from build123d import *

# Parameters (mm, degrees)
EXTRUDE_THIN1_DEPTH      = 10
EXTRUDE_THIN1_DEPTH_BACK = 25
SKETCH1_R                = 27.5
SKETCH1_R_2              = 22.5
CUT_EXTRUDE1_REACH       = 68.38
CUT_EXTRUDE1_END_RADIUS  = 22.5
SKETCH2_R                = 3.5
BOSS_EXTRUDE1_START      = -5
SKETCH3_R                = 22.5
BOSS_EXTRUDE1_DEPTH      = 5


with BuildPart() as part:
    # Sketch1 → Extrude-Thin1 (new, two sides: drawn at the far end of the back side and taken through both)
    with BuildSketch(Plane(origin=(0, 0, 0), x_dir=(1, 0, 0), z_dir=(0, 1, 0)).offset(-EXTRUDE_THIN1_DEPTH_BACK)):
        Circle(SKETCH1_R)
        Circle(SKETCH1_R_2, mode=Mode.SUBTRACT)
    extrude(amount=EXTRUDE_THIN1_DEPTH + EXTRUDE_THIN1_DEPTH_BACK)

    # Cut-Extrude1: up to this cylinder (the profile starts outside it)
    cut_extrude1_end = Plane(origin=(0, 0, 0), z_dir=(0, 1, 0)) * Cylinder(CUT_EXTRUDE1_END_RADIUS, 182.76, mode=Mode.PRIVATE)
    # Sketch2 → Cut-Extrude1 (cut, up to the surface)
    with BuildSketch(Plane.XY.offset(27.5), mode=Mode.PRIVATE) as cut_extrude1_sk1:
        with Locations(Location((0, 0, 0), (0, 0, 270))):
            Circle(SKETCH2_R)
    cut_extrude1_tool1 = extrude(cut_extrude1_sk1.sketch, amount=-CUT_EXTRUDE1_REACH, mode=Mode.PRIVATE) - cut_extrude1_end
    cut_extrude1 = cut_extrude1_tool1.solids().sort_by_distance((0, 0, 27.5))[0]
    add(cut_extrude1, mode=Mode.SUBTRACT)

    # Mirror1: Cut-Extrude1 across plane
    add(cut_extrude1.mirror(Plane.XY), mode=Mode.SUBTRACT)

    # Sketch3 → Boss-Extrude1 (add)
    with BuildSketch(Plane.XZ.offset(25).offset(BOSS_EXTRUDE1_START)):
        with Locations(Location((0, 0, 0), (0, 0, 90))):
            Circle(SKETCH3_R)
    extrude(amount=BOSS_EXTRUDE1_DEPTH)


solid = part.part
Can you work these out from the model? Positions are in its coordinate system, mm. A direction names the side the tool comes from. Round coordinates to 2 decimals unless told otherwise and drop trailing zeros. Order: outer loops, then holes, each group sorted by start corner. A loop starts at its lowest first (then second) coordinate and runs counter-clockwise, first axis right, second up. Notation, with made-up numbers: (-16, 23.25) - (26, 23.25) arc R25 cw to (26, 52.25) - close; hole circle Ø8 at (49, 82). An arc over 180 degrees is marked (long way). Answer in a Markdown table with one row per item.
(1) If we mould it in two halves opening along X, with no side actions, what happens to faces 3 (the face through (-5.961, -7.745, 26.846)), 4 (the face through (-3.417, 0.759, -24.9)), 5 (the face through (-23, 10, 0))? For each: released by +X, released by -X, zero draft, split by the parting line, or undercut.
From the geometry:
| item | result |
|---|---|
| face 3 | split by the parting line |
| face 4 | undercut |
| face 5 | zero draft |
(2) Suppose I cut it at B-B, the plane z = 0. Please give me the cut outline in (x, y), plus the area to 3 significant figures.
From the geometry:
| item | result |
|---|---|
| outline | (-27.5, -25) - (27.5, -25) - (27.5, 10) - (22.5, 10) - (22.5, -20) - (-22.5, -20) - (-22.5, 10) - (-27.5, 10) - close |
| area | 575 mm2 |
(3) Please list where these lines run through material, in increasing order: L1, parallel to Y at x = 0, z = -24; L2, parallel to Z at x = 0, y = -6; L3, parallel to X at y = -10, z = -14. Write a range as from..to.
From the geometry:
| item | result |
|---|---|
| L1 | y = -25..-3.5, 3.5..10 |
| L2 | z = -27.5..-22.5, 22.5..27.5 |
| L3 | x = -23.67..-17.61, 17.61..23.67 |
(4) Suppose I cut it at D-D, the plane y = -11. Please give me the cut outline in (x, z), plus the area to 3 significant figures.
From the geometry:
| item | result |
|---|---|
| outline | circle Ø55 at (0, 0); hole circle Ø45 at (0, 0) |
| area | 785 mm2 |
(5) For P1, Ø1, axis at y = -6.5, z = -13, coming from the +X side; P2, Ø2, axis at x = 10.5, z = 1.5, coming from the +Y side; P3, Ø8, axis at y = -15, z = 16.5, coming from the -X side; P4, Ø11, axis at x = 0, y = 0, coming from the -Z side, each with a flat end and sliding along its axis, tell me the tip position at first contact or that it passes through.
From the geometry:
| item | result |
|---|---|
| P1 | stops at x = 24.49 |
| P2 | stops at y = -20 |
| P3 | stops at x = -24.49 |
| P4 | stops at z = -27.5 |
(6) Which directions (+Z, -Z, +X, -X, +Y, -Y) give clear straight access to the entire face, cutting with the end or side of a thin tool? Please do faces 1 (the face through (-1.341, -3.233, 24.9)), 2 (the face through (-4.878, -5.21, 21.965)).
From the geometry:
| item | result |
|---|---|
| face 1 | +Z, -Z |
| face 2 | +Y |
(7) Suppose I cut it at A-A, the plane x = 0. Please give me the cut outline in (y, z), plus the area to 3 significant figures.
From the geometry:
| item | result |
|---|---|
| outline | (-25, -27.5) - (-3.5, -27.5) - (-3.5, -22.5) - (-20, -22.5) - (-20, 22.5) - (-3.5, 22.5) - (-3.5, 27.5) - (-25, 27.5) - close; (3.5, -27.5) - (10, -27.5) - (10, -22.5) - (3.5, -22.5) - close; (3.5, 22.5) - (10, 22.5) - (10, 27.5) - (3.5, 27.5) - close |
| area | 505 mm2 |
(8) Suppose I cut it at C-C, the plane y = 0. Please give me the cut outline in (x, z).
From the geometry:
| item | result |
|---|---|
| outline | (-3.5, -27.28) - (-3.5, -22.23) arc R22.5 cw to (-3.5, 22.23) - (-3.5, 27.28) arc R27.5 ccw to start; (3.5, -27.28) arc R27.5 ccw to (3.5, 27.28) - (3.5, 22.23) arc R22.5 cw to (3.5, -22.23) - close |
